Geometry check sheet. Reference: the model listing, model coordinates, mm. A direction names the side the tool comes from. Round coordinates to 2 decimals unless told otherwise and drop trailing zeros. Loops run counter-clockwise (first coordinate to the right, second up) from the corner with the lowest first, then second, coordinate; pieces in that order, holes last. Notation, with made-up numbers: (87, 62) - (129, 62) arc R8 cw to (129, 77) - close; hole circle Ø5 at (53.5, -18.5). An arc over 180 degrees is marked (long way). Write item = value, one per line.
```python
from build123d import *

# Parameters (mm, degrees)
BOSS_EXTRUDE1_DEPTH = 2.794
SKETCH2_R           = 2
SKETCH2_R_2         = 0.8
SKETCH2_W           = 1.5875
SKETCH2_H           = 6.35
CUT_EXTRUDE1_DEPTH  = 157.484941985
FILLET1_R           = 10.16


with BuildPart() as part:
    # Sketch1 → Boss-Extrude1 (new body)
    with BuildSketch(Plane(origin=(85.09, 0, 0), x_dir=(0, 0, -1), z_dir=(1, 0, 0))):
        with BuildLine():
            Line((-64.730392893, 73.865929303), (-64.730392893, 44.496360983))
            Line((-64.730392893, 44.496360983), (-13.648686174, 44.496360983))
            Line((-13.648686174, 44.496360983), (-6.823686174, 51.321360983))
            Line((-6.823686174, 51.321360983), (20.646158347, 51.321360983))
            Line((20.646158347, 51.321360983), (20.646158347, 44.496360983))
            Line((20.646158347, 44.496360983), (23.440158347, 44.496360983))
            Line((23.440158347, 44.496360983), (23.440158347, 38.146360983))
            Line((23.440158347, 38.146360983), (20.646158347, 38.146360983))
            Line((20.646158347, 38.146360983), (20.646158347, 31.796360983))
            Line((20.646158347, 31.796360983), (14.296158347, 31.796360983))
            Line((14.296158347, 31.796360983), (14.296158347, 29.002360983))
            Line((14.296158347, 29.002360983), (7.946158347, 29.002360983))
            Line((7.946158347, 29.002360983), (7.946158347, 31.796360983))
            Line((7.946158347, 31.796360983), (-35.003841653, 31.796360983))
            Line((-35.003841653, 31.796360983), (-35.003841653, 29.002360983))
            Line((-35.003841653, 29.002360983), (-41.353841653, 29.002360983))
            Line((-41.353841653, 29.002360983), (-41.353841653, 31.796360983))
            Line((-41.353841653, 31.796360983), (-69.928841653, 31.796360983))
            Line((-69.928841653, 31.796360983), (-69.928841653, 29.002360983))
            Line((-69.928841653, 29.002360983), (-76.278841653, 29.002360983))
            Line((-76.278841653, 29.002360983), (-76.278841653, 31.796360983))
            Line((-76.278841653, 31.796360983), (-82.628841653, 31.796360983))
            Line((-82.628841653, 31.796360983), (-82.628841653, 34.971360983))
            Line((-82.628841653, 34.971360983), (-85.422841653, 34.971360983))
            Line((-85.422841653, 34.971360983), (-85.422841653, 41.321360983))
            Line((-85.422841653, 41.321360983), (-82.628841653, 41.321360983))
            Line((-82.628841653, 41.321360983), (-82.628841653, 52.433860983))
            Line((-82.628841653, 52.433860983), (-85.422841653, 52.433860983))
            Line((-85.422841653, 52.433860983), (-85.422841653, 58.783860983))
            Line((-85.422841653, 58.783860983), (-82.628841653, 58.783860983))
            Line((-82.628841653, 58.783860983), (-82.628841653, 65.133860983))
            Line((-82.628841653, 65.133860983), (-77.61007114, 99.048207683))
            ThreePointArc((-77.61007114, 99.048207683), (-77.197997978, 100.104395563), (-76.367434478, 100.876082938))
            Line((-76.367434478, 100.876082938), (-74.680762236, 101.849883611))
            Line((-74.680762236, 101.849883611), (-68.330762236, 90.851360983))
            Line((-68.330762236, 90.851360983), (-65.911087258, 92.248360983))
            Line((-65.911087258, 92.248360983), (-72.261087258, 103.246883611))
            Line((-72.261087258, 103.246883611), (-68.96153047, 105.151883611))
            ThreePointArc((-68.96153047, 105.151883611), (-67.034130095, 105.405630684), (-65.491825944, 104.222179085))
            Line((-65.491825944, 104.222179085), (-61.681825944, 97.623065508))
            ThreePointArc((-61.681825944, 97.623065508), (-60.139521793, 96.439613909), (-58.212121418, 96.693360983))
            Line((-58.212121418, 96.693360983), (-28.956051228, 113.584360983))
            ThreePointArc((-28.956051228, 113.584360983), (-27.772599629, 115.126665134), (-28.026346702, 117.054065508))
            Line((-28.026346702, 117.054065508), (-31.836346702, 123.653179085))
            ThreePointArc((-31.836346702, 123.653179085), (-32.090093775, 125.58057946), (-30.906642177, 127.122883611))
            Line((-30.906642177, 127.122883611), (-27.607085388, 129.027883611))
            Line((-27.607085388, 129.027883611), (-21.257085388, 118.029360983))
            Line((-21.257085388, 118.029360983), (-18.83741041, 119.426360983))
            Line((-18.83741041, 119.426360983), (-25.18741041, 130.424883611))
            Line((-25.18741041, 130.424883611), (-24.637484279, 130.742383611))
            ThreePointArc((-24.637484279, 130.742383611), (-22.710083904, 130.996130684), (-21.167779753, 129.812679085))
            Line((-21.167779753, 129.812679085), (-13.547779753, 116.614451931))
            ThreePointArc((-13.547779753, 116.614451931), (-12.786538533, 110.832250808), (-16.33689333, 106.205338355))
            Line((-16.33689333, 106.205338355), (-60.920392893, 80.46504288))
            ThreePointArc((-60.920392893, 80.46504288), (-63.70950647, 77.675929303), (-64.730392893, 73.865929303))
        make_face()
    extrude(amount=BOSS_EXTRUDE1_DEPTH)

    # Sketch2 → Cut-Extrude1 (cut, through all)
    with BuildSketch(Plane(origin=(87.884, 0, 0), x_dir=(0, 0, -1), z_dir=(1, 0, 0))):
        with Locations((11.471158347, 43.146360983)):
            Circle(SKETCH2_R)
        with Locations((15.971158347, 43.146360983)):
            Circle(SKETCH2_R_2)
        with Locations((6.971158347, 43.146360983)):
            Circle(SKETCH2_R_2)
        Polygon((-24.575557246, 36.901889269), (-29.065685306, 41.392017329), (-31.041341653, 39.416360983), (-26.551213592, 34.926232922), align=None)
        with Locations((-78.660091653, 52.433860983)):
            Rectangle(SKETCH2_W, SKETCH2_H)
        Polygon((-38.682130644, 97.41042469), (-33.18286933, 100.58542469), (-34.57986933, 103.005099669), (-40.079130644, 99.830099669), align=None)
    extrude(amount=-CUT_EXTRUDE1_DEPTH, mode=Mode.SUBTRACT)

    # Fillet1
    fillet1_edges = [part.edges().sort_by_distance(p)[0] for p in [
        (86.487, 44.496360983, 64.730392893),
        (86.487, 44.496360983, 13.648686174),
        (86.487, 51.321360983, 6.823686174),
    ]]
    fillet(fillet1_edges, radius=FILLET1_R)


solid = part.part
```
(1) Section check A-A (x = 85.55). State how many separate pieces and enclosed holes the cut face has, then the cut area to 3 significant figures.
Answers follow:
separate_pieces = 1
enclosed_holes = 6
area = 3,390 mm²
(2) Set-up check for faces 4 (the flat face through (86, 52.434, 84)), 5 (the flat face through (86.47, 91.54, 67.14)), 6 (the flat face through (86, 31.796, 13)), 7 (the flat face through (87.884, 42, 39)), 8 (the flat face through (86, 44.496, -22)): record each of +Z, -Z, +X, -X, +Y, -Y from which the full face is reachable in a straight line by a thin tool's end or side.
Answers follow:
face_4 = +Z, +X, -X
face_5 = +X, -X
face_6 = +X, -X, -Y
face_7 = +Z, -Z, +X, +Y, -Y
face_8 = -Z, +X, -X, +Y
(3) Section check C-C (z = 8.5). Enter the section's corners in (x, y), then the cut area to 3 significant figures.
Answers follow:
outline = (85.09, 31.8) - (87.88, 31.8) - (87.88, 49.44) - (85.09, 49.44) - close
area = 49.3 mm²
(4) Scan lines: L1, parallel to Z at x = 87, y = 43; L2, parallel to Y at x = 85.7, z = 2.5; L3, parallel to Y at x = 87.8, z = 30. Record each from-to range of solid material in increasing order. Write a range as [from, to].
Answers follow:
L1 = [-23.44, -16.76], [-15.18, -13.47], [-9.48, -7.76], [-6.18, 82.63]
L2 = [31.8, 51.32]
L3 = [31.8, 38.38], [40.46, 44.5], [98.32, 112.98], [120.47, 127.65]
(5) Gauge pin test, flat ends, axial feed: pin 1 (1.4 mm diameter, centred on x = 87, z = 3.5, fed in from -Y); pin 2 (1.4 mm diameter, centred on x = 87, z = 83.5, fed in from -Y); pin 3 (1.4 mm diameter, centred on y = 43.15, z = -15.97, fed in from -X); pin 4 (0.8 mm diameter, centred on x = 87, z = -21.5, fed in from -Y). Record the tip position at first contact, or that the pin passes through.
Answers follow:
pin_1 = 31.8
pin_2 = 34.97
pin_3 = through
pin_4 = 38.15
(6) Section check B-B (y = 115). Enter the section's corners in (x, z).
Answers follow:
outline = (85.09, 12.85) - (87.88, 12.85) - (87.88, 27.81) - (85.09, 27.81) - close
(7) Mould release check, pull along Z, two halves, no side actions. Record for faces 1 (the flat face through (86, 29.002, 38)), 2 (the flat face through (86, 35, -20.646)), 3 (the flat face through (86, 30, 41.354)): pulls with the +Z half, pulls with the -Z half, needs draft (parallel to the pull), parting line crosses it, or undercut.
Answers follow:
face_1 = needs draft
face_2 = pulls with the -Z half
face_3 = undercut
